from build123d import *

# Parameters (mm, degrees)
SKETCH2_R           = 57.15
BOSS_EXTRUDE1_DEPTH = 9.525


with BuildPart() as part:
    # Sketch1 → Revolve1 (revolve)
    with BuildSketch(Plane.XY):
        Polygon((-30.1625, -57.15), (30.1625, -57.15), (30.1625, 0), (20.6375, 0), (20.6375, -51.1302), (-30.1625, -51.1302), align=None)
    revolve(axis=Axis((-30.1625, 0, 0), (1, 0, 0)))

    # Sketch2 → Boss-Extrude1 (add)
    with BuildSketch(Plane(origin=(30.1625, 0, 0), x_dir=(0, 0, -1), z_dir=(1, 0, 0))):
        Polygon((-24.001087105, 57.94375), (-57.94375, 24.001087105), (-57.94375, -24.001087105), (-24.001087105, -57.94375), (24.001087105, -57.94375), (57.94375, -24.001087105), (57.94375, 24.001087105), (24.001087105, 57.94375), align=None)
        Circle(SKETCH2_R, mode=Mode.SUBTRACT)
    extrude(amount=-BOSS_EXTRUDE1_DEPTH)


solid = part.part
CAD build for the part. Positions are in the model's coordinates, mm. A direction names the side the tool comes from. Coordinates: 2 decimals unless noted, no trailing zeros. Order: outer loops, then holes, each group sorted by start corner. A loop starts at its lowest first (then second) coordinate and runs counter-clockwise, first axis right, second up.
Item 1: Band-saw the part on B-B on z = 0. List the corners of the cut face in (x, y).
Check sheet entries:
outline: (-30.16, -57.15) - (20.64, -57.15) - (20.64, -57.94) - (30.16, -57.94) - (30.16, 57.94) - (20.64, 57.94) - (20.64, 57.15) - (-30.16, 57.15) - (-30.16, 51.13) - (20.64, 51.13) - (20.64, -51.13) - (-30.16, -51.13) - close
Item 2: Pin check, flat tips, straight feed: pin 1 Ø2 at (x, y) = (14.5, -37) entering from +Z; pin 2 Ø2 at (y, z) = (-31.5, 11) entering from -X; pin 3 Ø2 at (x, y) = (-19.5, -31.5) entering from -Z. Stop position of each tip, or through.
Check sheet entries:
pin 1: stops at z = 44.39
pin 2: stops at x = 20.64
pin 3: stops at z = -48.33
Item 3: Band-saw the part on D-D on x = 5.5. List the corners of the cut face in (y, z), plus the area to 3 significant figures.
Check sheet entries:
outline: circle Ø114.3 at (0, 0); hole circle Ø102.26 at (0, 0)
area: 2,050 mm2
Item 4: Two-plate mould, pull along Y, no slides. Class faces 3 (the face through (25.467, -41.21, -40.735)), 4 (the face through (25, 0, -57.944)), 5 (the face through (20.637, -1, -1)), 6 (the face through (25, 57.944, 0)): +Y half, -Y half, draft (parallel to the pull), parting line (faces both ways), or undercut.
Check sheet entries:
face 3: -Y half
face 4: draft
face 5: undercut
face 6: +Y half
Item 5: Drill centre lines: L1, parallel to Z at x = -17, y = 0; L2, parallel to X at y = 42.5, z = -22.5. Where is each one in solid material? Low to high.
Check sheet entries:
L1: z = -57.15 to -51.13, 51.13 to 57.15
L2: x = 20.64 to 30.16
Item 6: 3-axis set-ups, long thin cutter, end or side, ignore diameter. For faces 1 (the face through (-5.12, -48.77, -15.36)), 2 (the face through (25, 0, 57.944)): which of +Z, -Z, +X, -X, +Y, -Y reach the whole face in a straight line?
Check sheet entries:
face 1: -X
face 2: +Z, +X, -X, +Y, -Y
Item 7: Band-saw the part on A-A on x = 25.5. List the corners of the cut face in (y, z), plus the area to 3 significant figures.
Check sheet entries:
outline: (-57.94, -24) - (-24, -57.94) - (24, -57.94) - (57.94, -24) - (57.94, 24) - (24, 57.94) - (-24, 57.94) - (-57.94, 24) - close
area: 11,100 mm2
